from build123d import *

# Parameters (mm, degrees)
SKETCH1_R           = 1.5
BOSS_EXTRUDE1_DEPTH = 8
SKETCH2_R           = 4
SKETCH2_R_2         = 1.5
BOSS_EXTRUDE2_DEPTH = 2
SKETCH3_R           = 4
SKETCH3_R_2         = 2.75
BOSS_EXTRUDE3_DEPTH = 3
CUT_EXTRUDE1_DEPTH  = 3


with BuildPart() as part:
    # Sketch1 → Boss-Extrude1 (new body)
    with BuildSketch(Plane(origin=(0, 0, 0), x_dir=(1, 0, 0), z_dir=(0, 1, 0))):
        with BuildLine():
            Line((-7.5, 11.932713059), (-7.5, 0))
            ThreePointArc((-7.5, 0), (0, -7.5), (7.5, 0))
            Line((7.5, 0), (7.5, 11.932713059))
            ThreePointArc((7.5, 11.932713059), (7.452991921, 14.998558127), (7.31201188, 18.061520806))
            ThreePointArc((7.31201188, 18.061520806), (7.564401673, 21.22883688), (8.315200992, 24.31621313))
            ThreePointArc((8.315200992, 24.31621313), (10.803384698, 38.546346738), (9.119465085, 52.893896195))
            Line((9.119465085, 52.893896195), (4, 72))
            Line((4, 72), (4, 80))
            Line((4, 80), (-4, 80))
            Line((-4, 80), (-4, 72))
            Line((-4, 72), (-9.119465085, 52.893896195))
            ThreePointArc((-9.119465085, 52.893896195), (-10.803384698, 38.546346738), (-8.315200992, 24.31621313))
            ThreePointArc((-8.315200992, 24.31621313), (-7.564401673, 21.22883688), (-7.31201188, 18.061520806))
            ThreePointArc((-7.31201188, 18.061520806), (-7.452991921, 14.998558127), (-7.5, 11.932713059))
        make_face()
        with Locations(Location((0, 0, 0), (0, 0, 270))):
            Circle(SKETCH1_R, mode=Mode.SUBTRACT)
        with BuildLine():
            ThreePointArc((-3.28125, 22.259456382), (-4.983963759, 23.524670141), (-3.71875, 25.2273839))
            ThreePointArc((-3.71875, 25.2273839), (0, 25.5), (3.71875, 25.2273839))
            ThreePointArc((3.71875, 25.2273839), (4.983963759, 23.524670141), (3.28125, 22.259456382))
            ThreePointArc((3.28125, 22.259456382), (0, 22.5), (-3.28125, 22.259456382))
        make_face(mode=Mode.SUBTRACT)
    extrude(amount=BOSS_EXTRUDE1_DEPTH)

    # Sketch2 → Boss-Extrude2 (add)
    with BuildSketch(Plane(origin=(0, 8, 0), x_dir=(1, 0, 0), z_dir=(0, 1, 0))):
        with Locations(Location((0, 0, 0), (0, 0, 270))):
            Circle(SKETCH2_R)
        with Locations(Location((0, 0, 0), (0, 0, 270))):
            Circle(SKETCH2_R_2, mode=Mode.SUBTRACT)
    extrude(amount=BOSS_EXTRUDE2_DEPTH)

    # Sketch3 → Boss-Extrude3 (add)
    with BuildSketch(Plane(origin=(0, 10, 0), x_dir=(1, 0, 0), z_dir=(0, 1, 0))):
        with Locations(Location((0, 0, 0), (0, 0, 270))):
            Circle(SKETCH3_R)
        with Locations(Location((0, 0, 0), (0, 0, 270))):
            Circle(SKETCH3_R_2, mode=Mode.SUBTRACT)
    extrude(amount=BOSS_EXTRUDE3_DEPTH)

    # Sketch4 → Cut-Extrude1 (cut)
    with BuildSketch(Plane(origin=(0, 8, 0), x_dir=(1, 0, 0), z_dir=(0, 1, 0))):
        with BuildLine():
            ThreePointArc((3.098958333, 21.022819917), (6.220600225, 23.342378475), (3.901041667, 26.464020366))
            ThreePointArc((3.901041667, 26.464020366), (0, 26.75), (-3.901041667, 26.464020366))
            ThreePointArc((-3.901041667, 26.464020366), (-6.220600225, 23.342378475), (-3.098958333, 21.022819917))
            ThreePointArc((-3.098958333, 21.022819917), (0, 21.25), (3.098958333, 21.022819917))
        make_face()
    extrude(amount=-CUT_EXTRUDE1_DEPTH, mode=Mode.SUBTRACT)


solid = part.part
Check sheet for the modelled part. Datum: model origin and axes. Units: mm. A direction names the side the tool comes from. Give positions to 0.01 mm unless a question says otherwise; leave off trailing zeros. Loops run counter-clockwise (first coordinate to the right, second up) from the corner with the lowest first, then second, coordinate; pieces in that order, holes last. Notation, with made-up numbers: M 8,69 L 34,69 A23 ccw 34,105 Z; hole C -15.75,-22.75 d2. An arc over 180 degrees is marked long. Answer as a JSON object with one key per item and string values. Group by question number.
Q1. Access from +Z, -Z, +X, -X, +Y, -Y to the whole of each face (thin tool, end or side, straight path). Record for faces 5 (the cylindrical face through (7.557, 3.944, -21.185)), 6 (the flat face through (4, 4, -76)), 7 (the flat face through (-6.524, 3.944, -62.581)), 8 (the cylindrical face through (-2.685, 11.479, -0.596)), 9 (the cylindrical face through (-7.57, 3.94, -21.27)).
Q2. Go/stop test with flat-tipped pins: P1, Ø1.7, axis at x = 3, z = -24.5, coming from the +Y side; P2, Ø4, axis at y = 4.5, z = -7.5, coming from the +X side; P3, Ø4, axis at y = 3, z = -5.5, coming from the -X side. Record where each tip stops, or that it passes through.
Q3. Material ranges on line 1 along X through (y, z) = (11.5, 0); line 2 along Z through (x, y) = (1, 1); line 3 along Y through (x, z) = (-5, -32), recorded low to high. Write a range as [from, to].
Q4. Release check for a two-part mould opening along Z. For faces 1 (the flat face through (0, 0, -37)), 2 (the cylindrical face through (0.05, 6.52, -26.75)), 3 (the cylindrical face through (0, 2.5, -22.5)), 4 (the cylindrical face through (-3.905, 10.465, -0.867)) record: released by +Z, released by -Z, zero draft, split by the parting line, or undercut.
Q5. Cross-section at C-C on z = -62. Record the cut outline in (x, y).
Q6. Cross-section at A-A on y = 6. Record the cut outline in (x, z), then the cut area to 3 significant figures.
Q7. Cross-section at D-D on z = -19.5. Record the cut outline in (x, y).
Q8. Cross-section at B-B on x = 0. Record the cut outline in (y, z).
Evaluation:
{
 "1": {"face 5": "+X, +Y, -Y", "face 6": "-Z, +X, +Y, -Y", "face 7": "-Z, -X, +Y, -Y", "face 8": "+Y", "face 9": "-X, +Y, -Y"},
 "2": {"P1": "stops at y = 5", "P2": "stops at x = 7.5", "P3": "stops at x = -7.5"},
 "3": {"line 1": "x = [-4, -2.75], [2.75, 4]", "line 2": "z = [-80, -25.48], [-22.48, -1.12], [1.12, 7.43]", "line 3": "y = [0, 8]"},
 "4": {"face 1": "zero draft", "face 2": "undercut", "face 3": "undercut", "face 4": "split by the parting line"},
 "5": {"outline": "M -6.68,0 L 6.68,0 L 6.68,8 L -6.68,8 Z"},
 "6": {"outline": "M -9.12,-52.89 L -4,-72 L -4,-80 L 4,-80 L 4,-72 L 9.12,-52.89 A50 ccw 8.32,-24.32 A20 cw 7.31,-18.06 A100 ccw 7.5,-11.93 L 7.5,0 A7.5 ccw -7.5,0 L -7.5,-11.93 A100 ccw -7.31,-18.06 A20 cw -8.32,-24.32 A50 ccw Z; hole M -3.9,-26.46 A26.75 ccw 3.9,-26.46 A2.75 ccw 3.1,-21.02 A21.25 cw -3.1,-21.02 A2.75 ccw Z; hole C 0,0 d3", "area": "1,280 mm2"},
 "7": {"outline": "M -7.36,0 L 7.36,0 L 7.36,8 L -7.36,8 Z"},
 "8": {"outline": "M 0,-80 L 8,-80 L 8,-26.75 L 5,-26.75 L 5,-25.5 L 0,-25.5 Z; M 0,-22.5 L 5,-22.5 L 5,-21.25 L 8,-21.25 L 8,-4 L 13,-4 L 13,-2.75 L 10,-2.75 L 10,-1.5 L 0,-1.5 Z; M 0,1.5 L 10,1.5 L 10,2.75 L 13,2.75 L 13,4 L 8,4 L 8,7.5 L 0,7.5 Z"}
}
